Verification items for the finished model (mm, model axes). A direction names the side the tool comes from. Give positions to 0.01 mm unless a question says otherwise; leave off trailing zeros. Order: outer loops, then holes, each group sorted by start corner. A loop starts at its lowest first (then second) coordinate and runs counter-clockwise, first axis right, second up. Notation, with made-up numbers: (62, -9.75) -> (109, -9.75) arc R11 cw to (109, 3.25) -> close; hole circle Ø10 at (85.5, 19.5). An arc over 180 degrees is marked (long way). Return JSON: item names as keys, results as strings. Group by question number.
(1) Depth check by flat-ended pin: pin 1 Ø5 at (x, z) = (-22, -39.5) entering from +Y (3 decimals); pin 2 Ø11.5 at (x, z) = (-101.5, -10.5) entering from -Y; pin 3 Ø1 at (y, z) = (11, -7.5) entering from -X; pin 4 Ø5 at (y, z) = (3, -33) entering from +X. Enter the tip coordinate at first touch or a pass-through.
(2) Cross-section at C-C on z = -17. Enter the section's corners in (x, y), then the cut area to 3 significant figures.
(3) Cross-section at B-B on x = -19. Enter the section's corners in (y, z).
(4) Tool access check on faces 1 (the face through (-92, 5, -30)), 2 (the face through (-89.455, -12.64, -28.49)), 3 (the face through (5, 0, -44)). Record the directions out of +Z, -Z, +X, -X, +Y, -Y that give a thin tool (end or side, any length) a straight path to the whole face; none if there is none.
(5) Cross-section at A-A on y = -11. Enter the section's corners in (x, z), then the cut area to 3 significant figures.
(6) Thickness scan on line 1 along Z through (x, y) = (77, 19.45); line 2 along X through (y, z) = (18.6, -47); line 3 along Z through (x, y) = (-39.5, -14). Record the ranges inside material, lowest first.
from build123d import *

# Parameters (mm, degrees)
BOSS_EXTRUDE1_DEPTH = 22.5
SKETCH2_R           = 1.5
CUT_EXTRUDE1_DEPTH  = 5
FILLET1_R           = 2
SKETCH3_W           = 35
SKETCH3_H           = 20
CUT_EXTRUDE2_DEPTH  = 10
SKETCH6_W           = 44
SKETCH6_H           = 45
CUT_EXTRUDE3_DEPTH  = 123.907485533


with BuildPart() as part:
    # Sketch1 → Boss-Extrude1 (new, symmetric)
    with BuildSketch(Plane(origin=(0, 0, 0), x_dir=(1, 0, 0), z_dir=(0, 1, 0))):
        Polygon((-110, 0), (-80, 50), (80, 50), (110, 0), (103, 0), (76.6, 44), (-76.6, 44), (-103, 0), align=None)
    extrude(amount=BOSS_EXTRUDE1_DEPTH, both=True)

    # Sketch2 → Cut-Extrude1 (cut)
    with BuildSketch(Plane(origin=(0, 22.5, 0), x_dir=(1, 0, 0), z_dir=(0, 1, 0))):
        with Locations(Location((-98.701428863, 13, 0), (0, 0, 270))):
            Circle(SKETCH2_R)
        with Locations(Location((-77, 47, 0), (0, 0, 270))):
            Circle(SKETCH2_R)
        with Locations(Location((-7, 47, 0), (0, 0, 270))):
            Circle(SKETCH2_R)
        with Locations(Location((7, 47, 0), (0, 0, 90))):
            Circle(SKETCH2_R)
        with Locations(Location((77, 47, 0), (0, 0, 90))):
            Circle(SKETCH2_R)
        with Locations(Location((98.701428863, 13, 0), (0, 0, 90))):
            Circle(SKETCH2_R)
    extrude(amount=-CUT_EXTRUDE1_DEPTH, mode=Mode.SUBTRACT)

    # Fillet1
    fillet1_edges = [part.edges().sort_by_distance(p)[0] for p in [
        (-80, 0, -50),
        (80, 0, -50),
    ]]
    fillet(fillet1_edges, radius=FILLET1_R)

    # Sketch3 → Cut-Extrude2 (cut)
    with BuildSketch(Plane(origin=(-80.882352941, 0, -48.529411765), x_dir=(-0.5144957554275265, 0, 0.8574929257125443), z_dir=(-0.8574929257125443, 0, -0.5144957554275265))):
        with Locations((39.094533097, -12.5)):
            Rectangle(SKETCH3_W, SKETCH3_H)
    extrude(amount=-CUT_EXTRUDE2_DEPTH, mode=Mode.SUBTRACT)

    # Sketch6 → Cut-Extrude3 (cut, through all)
    with BuildSketch(Plane(origin=(0, 0, 0), x_dir=(0, 0, -1), z_dir=(1, 0, 0))):
        with Locations((22, 0)):
            Rectangle(SKETCH6_W, SKETCH6_H)
    extrude(amount=CUT_EXTRUDE3_DEPTH, mode=Mode.SUBTRACT)


solid = part.part
Verdict:
{
 "1": {"pin 1": "through", "pin 2": "y = -2.5", "pin 3": "x = -105.8", "pin 4": "x = -81.7"},
 "2": {"outline": "(-99.8, -2.5) -> (-92.8, -2.5) -> (-92.8, 22.5) -> (-99.8, 22.5) -> close", "area": "175 mm²"},
 "3": {"outline": "(-22.5, -50) -> (22.5, -50) -> (22.5, -44) -> (-22.5, -44) -> close"},
 "4": {"face 1": "-Z, -X, +Y, -Y", "face 2": "+Z, -X, -Y", "face 3": "+Z, +X, +Y, -Y"},
 "5": {"outline": "(-91.99, -30.01) -> (-80.58, -49.03) arc R2 ccw to (-78.87, -50) -> (78.87, -50) arc R2 ccw to (80.58, -49.03) -> (83.6, -44) -> (-76.6, -44) -> (-86.85, -26.92) -> close", "area": "1,090 mm²"},
 "6": {"line 1": "-50 to -48.5, -45.5 to -44", "line 2": "-81.8 to -78.5, -75.5 to -8.5, -5.5 to 5.5, 8.5 to 75.5, 78.5 to 81.8", "line 3": "-50 to -44"}
}
